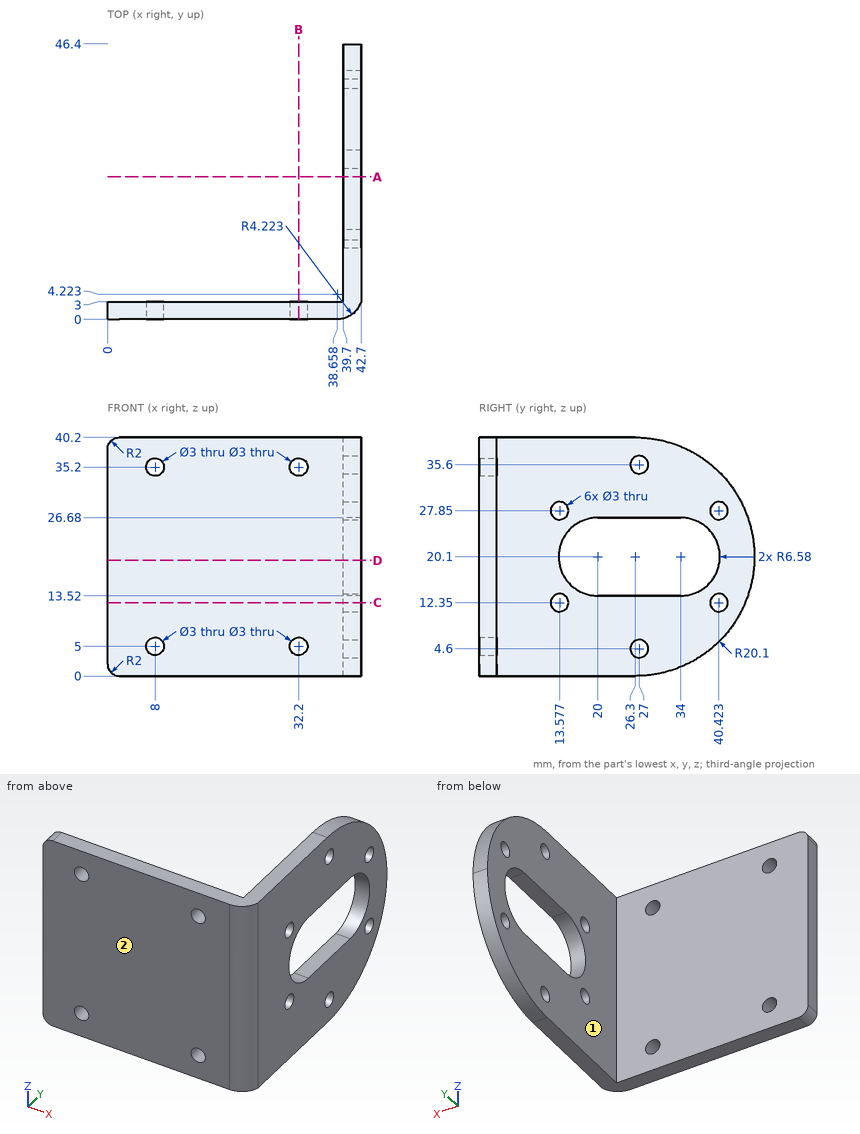
Input: dimensioned drawing with shaded views. Units: mm. Origin: part minimum x, y, z. A direction names the side the tool comes from. Coordinates: 2 decimals unless noted, no trailing zeros. Order: outer loops, then holes, each group sorted by start corner. A loop starts at its lowest first (then second) coordinate and runs counter-clockwise, first axis right, second up. Notation, with made-up numbers: M 88.5,-21.5 L 130.5,-21.5 A18 ccw 130.5,1.5 Z; hole C 64,8.5 d4. An arc over 180 degrees is marked long. Write each question's results on one line, items separated by ' | '. Start each with the question number.
Item 1: First-contact query: pin 1 Ø3.5 at (y, z) = (40.42, 27.85) entering from +X; pin 2 Ø5 at (x, z) = (32.2, 5) entering from +Y; pin 3 Ø10 at (x, y) = (30, 36.5) entering from -Z; pin 4 Ø5 at (y, z) = (17, 17) entering from -X. Flat tips, straight axial feed; report the tip coordinate or a pass-through.
Item 2: Line query: probe 1 along Z at (x, y) = (8, 1.2); probe 2 along Y at (x, z) = (40, 27); probe 3 along Y at (x, z) = (41, 27). Output: solid intervals per line, ascending.
Item 3: Set-up query: the marked faces 1 and 2. Return all of +Z, -Z, +X, -X, +Y, -Y with unobstructed straight access to the full face (end or side cutting, diameter ignored); none if empty.
Item 4: Cut plane C-C (z = 12.35). Return loops of the section in (x, y).
Item 5: Cut plane A-A (y = 24). Return loops of the section in (x, z).
Item 6: Cut plane B-B (x = 32.2). Return loops of the section in (y, z).
Item 7: Cut plane D-D (z = 19.5). Return loops of the section in (x, y).
Checked values:
1) pin 1: stops at x = 42.7 | pin 2: stops at y = 3 | pin 3: passes through | pin 4: stops at x = 39.7
2) probe 1: z = 0 to 3.5, 6.5 to 33.7, 36.7 to 40.2 | probe 2: y = 0.22 to 12.34, 14.81 to 39.19, 41.66 to 45.18 | probe 3: y = 0.71 to 12.34, 14.81 to 39.19, 41.66 to 45.18
3) face 1: +Z, -Z, -X, +Y | face 2: +Z, -Z, +X, -X, -Y
4) outline: M 0,0 L 38.66,0 A4.22 ccw 42.7,3 L 42.7,12.08 L 39.7,12.08 L 39.7,3 L 0,3 Z; M 39.7,15.08 L 42.7,15.08 L 42.7,38.92 L 39.7,38.92 Z; M 39.7,41.92 L 42.7,41.92 L 42.7,44.85 L 39.7,44.85 Z
5) outline: M 39.7,0 L 42.7,0 L 42.7,13.52 L 39.7,13.52 Z; M 39.7,26.68 L 42.7,26.68 L 42.7,40.2 L 39.7,40.2 Z
6) outline: M 0,0 L 3,0 L 3,3.5 L 0,3.5 Z; M 0,6.5 L 3,6.5 L 3,33.7 L 0,33.7 Z; M 0,36.7 L 3,36.7 L 3,40.2 L 0,40.2 Z
7) outline: M 0,0 L 38.66,0 A4.22 ccw 42.7,3 L 42.7,13.45 L 39.7,13.45 L 39.7,3 L 0,3 Z; M 39.7,40.55 L 42.7,40.55 L 42.7,46.39 L 39.7,46.39 Z
